CAD build for the part. Positions are in the model's coordinates, mm. A direction names the side the tool comes from. Round coordinates to 2 decimals unless told otherwise and drop trailing zeros. Order: outer loops, then holes, each group sorted by start corner. A loop starts at its lowest first (then second) coordinate and runs counter-clockwise, first axis right, second up. Notation, with made-up numbers: (55.25, 66.25) - (100.25, 66.25) arc R15 ccw to (100.25, 95.25) - close; hole circle Ø4 at (-38.5, 77.25). An arc over 180 degrees is marked (long way). Write item = value, one per line.
from build123d import *

# Parameters (mm, degrees)
SKETCH1_W           = 50.8
SKETCH1_H           = 111.125
BOSS_EXTRUDE1_DEPTH = 1.5
SKETCH2_W           = 9.525
SKETCH2_H           = 9.525
BOSS_EXTRUDE2_DEPTH = 3
CUT_EXTRUDE1_DEPTH  = 3
FILLET1_R           = 1.5875
SKETCH5_W           = 3
SKETCH5_H           = 6.35
BOSS_EXTRUDE3_DEPTH = 3


with BuildPart() as part:
    # Sketch1 → Boss-Extrude1 (new, symmetric)
    with BuildSketch(Plane(origin=(0, 34.29, 0), x_dir=(1, 0, 0), z_dir=(0, 1, 0))):
        with Locations((0, 120.65)):
            Rectangle(SKETCH1_W, SKETCH1_H)
    extrude(amount=BOSS_EXTRUDE1_DEPTH, both=True)

    # Sketch2 → Boss-Extrude2 (add)
    with BuildSketch(Plane(origin=(0, 35.79, 0), x_dir=(1, 0, 0), z_dir=(0, 1, 0))):
        with Locations((30.1625, 171.45)):
            Rectangle(SKETCH2_W, SKETCH2_H)
        with Locations((-30.1625, 171.45)):
            Rectangle(SKETCH2_W, SKETCH2_H)
        with Locations((30.1625, 120.65)):
            Rectangle(SKETCH2_W, SKETCH2_H)
        with Locations((-30.1625, 120.65)):
            Rectangle(SKETCH2_W, SKETCH2_H)
        with Locations((30.1625, 69.85)):
            Rectangle(SKETCH2_W, SKETCH2_H)
        with Locations((-30.1625, 69.85)):
            Rectangle(SKETCH2_W, SKETCH2_H)
    extrude(amount=-BOSS_EXTRUDE2_DEPTH)

    # Sketch4 → Cut-Extrude1 (cut)
    with BuildSketch(Plane(origin=(0, 35.79, 0), x_dir=(1, 0, 0), z_dir=(0, 1, 0))):
        Polygon((17.042345512, 169.8625), (-17.042345512, 169.8625), (0, 147.84947038), align=None)
        Polygon((-2.007654488, 145.25625), (-19.05, 167.26927962), (-19.05, 123.24322038), align=None)
        Polygon((19.05, 167.26927962), (2.007654488, 145.25625), (19.05, 123.24322038), align=None)
        Polygon((15.813313254, 122.2375), (0, 142.66302962), (-15.813313254, 122.2375), align=None)
        Polygon((-2.007654488, 96.04375), (-19.05, 118.05677962), (-19.05, 74.03072038), align=None)
        Polygon((15.813313254, 119.0625), (-15.813313254, 119.0625), (0, 98.63697038), align=None)
        Polygon((19.05, 74.03072038), (19.05, 118.05677962), (2.007654488, 96.04375), align=None)
        Polygon((17.042345512, 71.4375), (0, 93.45052962), (-17.042345512, 71.4375), align=None)
    extrude(amount=-CUT_EXTRUDE1_DEPTH, mode=Mode.SUBTRACT)

    # Fillet1
    fillet1_edges = [part.edges().sort_by_distance(p)[0] for p in [
        (15.813313254, 34.29, -122.2375),
        (-15.813313254, 34.29, -122.2375),
        (0, 34.29, -142.66302962),
        (15.813313254, 34.29, -119.0625),
        (0, 34.29, -98.63697038),
        (-15.813313254, 34.29, -119.0625),
        (17.042345512, 34.29, -71.4375),
        (-17.042345512, 34.29, -71.4375),
        (0, 34.29, -93.45052962),
        (-2.007654488, 34.29, -96.04375),
        (-19.05, 34.29, -74.03072038),
        (-19.05, 34.29, -118.05677962),
        (-2.007654488, 34.29, -145.25625),
        (-19.05, 34.29, -123.24322038),
        (-19.05, 34.29, -167.26927962),
        (19.05, 34.29, -123.24322038),
        (2.007654488, 34.29, -145.25625),
        (19.05, 34.29, -167.26927962),
        (0, 34.29, -147.84947038),
        (-17.042345512, 34.29, -169.8625),
        (17.042345512, 34.29, -169.8625),
        (19.05, 34.29, -118.05677962),
        (19.05, 34.29, -74.03072038),
        (2.007654488, 34.29, -96.04375),
        (34.925, 34.29, -65.0875),
        (34.925, 34.29, -74.6125),
        (25.4, 34.29, -74.6125),
        (-25.4, 34.29, -115.8875),
        (-25.4, 34.29, -125.4125),
        (-34.925, 34.29, -125.4125),
        (-34.925, 34.29, -115.8875),
        (34.925, 34.29, -115.8875),
        (34.925, 34.29, -125.4125),
        (25.4, 34.29, -125.4125),
        (25.4, 34.29, -115.8875),
        (-25.4, 34.29, -166.6875),
        (-34.925, 34.29, -176.2125),
        (-34.925, 34.29, -166.6875),
        (-25.4, 34.29, -74.6125),
        (-34.925, 34.29, -74.6125),
        (-34.925, 34.29, -65.0875),
        (34.925, 34.29, -166.6875),
        (34.925, 34.29, -176.2125),
        (25.4, 34.29, -166.6875),
    ]]
    fillet(fillet1_edges, radius=FILLET1_R)

    # Sketch5 → Boss-Extrude3 (add)
    with BuildSketch(Plane(origin=(0, 35.79, 0), x_dir=(1, 0, 0), z_dir=(0, 1, 0))):
        with Locations((36.425, 171.45)):
            Rectangle(SKETCH5_W, SKETCH5_H)
        with Locations((-36.425, 171.45)):
            Rectangle(SKETCH5_W, SKETCH5_H)
        with Locations((36.425, 120.65)):
            Rectangle(SKETCH5_W, SKETCH5_H)
        with Locations((-36.425, 120.65)):
            Rectangle(SKETCH5_W, SKETCH5_H)
        with Locations((36.425, 69.85)):
            Rectangle(SKETCH5_W, SKETCH5_H)
        with Locations((-36.425, 69.85)):
            Rectangle(SKETCH5_W, SKETCH5_H)
    extrude(amount=-BOSS_EXTRUDE3_DEPTH)


solid = part.part
(1) Drop flat-ended pins along their axis: pin 1 (1.5 mm diameter, centred on y = 34, z = -143.5, fed in from -X); pin 2 (2 mm diameter, centred on x = -6.5, z = -81, fed in from -Y); pin 3 (1.5 mm diameter, centred on x = -36, y = 34, fed in from +Z) (3 decimals); pin 4 (1.5 mm diameter, centred on x = 36.5, y = 34.5, fed in from -Z) (3 decimals). Give the stop position or say it passes through.
Solved:
pin_1 = -25.4
pin_2 = through
pin_3 = -66.675
pin_4 = -174.625
(2) Probe line 1 along Z through (x, y) = (-30.5, 35.65); line 2 along Z through (x, y) = (-1.5, 34.3); line 3 along X through (y, z) = (34.8, -164). List the from-to ranges inside material, lowest first.
Solved:
line_1 = -176.21 to -166.69, -125.41 to -115.89, -74.61 to -65.09
line_2 = -176.21 to -169.86, -149.79 to -140.73, -122.24 to -119.06, -100.57 to -91.51, -71.44 to -65.09
line_3 = -25.4 to -18.26, -16.67 to -12.5, 12.5 to 16.67, 18.26 to 25.4
(3) Pull direction Z, two halves, no side cores. Call faces 1 (the flat face through (-9.39, 34.31, -154.79)), 2 (the flat face through (36, 34, -174.625)), 3 (the flat face through (-37.925, 34, -171)): released by +Z, released by -Z, zero draft, split by the parting line, or undercut.
Solved:
face_1 = undercut
face_2 = released by -Z
face_3 = zero draft
(4) Band-saw the part on A-A on z = -89.5. List the corners of the cut face in (x, y), plus the area to 3 significant figures.
Solved:
outline = (-25.4, 32.79) - (-19.05, 32.79) - (-19.05, 35.79) - (-25.4, 35.79) - close; (-7.07, 32.79) - (-3.06, 32.79) - (-3.06, 35.79) - (-7.07, 35.79) - close; (3.06, 32.79) - (7.07, 32.79) - (7.07, 35.79) - (3.06, 35.79) - close; (19.05, 32.79) - (25.4, 32.79) - (25.4, 35.79) - (19.05, 35.79) - close
area = 62.2 mm²
(5) Band-saw the part on C-C on y = 33.65. Count the separate pieces of the cut face and the enclosed holes in it, plus the area to 3 significant figures.
Solved:
separate_pieces = 1
enclosed_holes = 8
area = 3,460 mm²
(6) Band-saw the part on B-B on x = -5. List the corners of the cut face in (y, z).
Solved:
outline = (32.79, -176.21) - (35.79, -176.21) - (35.79, -169.86) - (32.79, -169.86) - close; (32.79, -154.31) - (35.79, -154.31) - (35.79, -149.12) - (32.79, -149.12) - close; (32.79, -141.39) - (35.79, -141.39) - (35.79, -136.2) - (32.79, -136.2) - close; (32.79, -122.24) - (35.79, -122.24) - (35.79, -119.06) - (32.79, -119.06) - close; (32.79, -105.1) - (35.79, -105.1) - (35.79, -99.91) - (32.79, -99.91) - close; (32.79, -92.18) - (35.79, -92.18) - (35.79, -86.99) - (32.79, -86.99) - close; (32.79, -71.44) - (35.79, -71.44) - (35.79, -65.09) - (32.79, -65.09) - close
(7) Tool access for faces 4 (the flat face through (25.4, 34, -146)), 5 (the flat face through (-9.39, 34.31, -105.58)), 6 (the flat face through (-25.4, 34, -95)): list every direction of +Z, -Z, +X, -X, +Y, -Y with a clear straight run to the whole face (end or side of a thin tool).
Solved:
face_4 = +X, +Y, -Y
face_5 = +Y, -Y
face_6 = -X, +Y, -Y
